Model file for the job. Use its own axes, mm. Round coordinates to 2 decimals unless told otherwise and drop trailing zeros. Loops run counter-clockwise (first coordinate to the right, second up) from the corner with the lowest first, then second, coordinate; pieces in that order, holes last. Notation, with made-up numbers: M -10,1 L 32,1 A12 ccw 32,22 Z; hole C -23.75,-29.5 d8. An arc over 180 degrees is marked long. Use a Markdown table: item, result. Add a question column.
Item 1: Saw through at B-B on y = -31. Write the cut outline in (x, z), then the cut area to 3 significant figures.
Item 2: Saw through at D-D on y = -20. Write the cut outline in (x, z).
Item 3: Saw through at A-A on x = 85.5. Write the cut outline in (y, z).
Item 4: Two-plate mould, pull along Y, no slides. Class faces 1 (the flat face through (11, 1, 2)), 2 (the cylindrical face through (81.73, 30.35, 0.99)): +Y half, -Y half, draft (parallel to the pull), parting line (faces both ways), or undercut.
Item 5: Saw through at C-C on z = 1.1. Write the cut outline in (x, y), then the cut area to 3 significant figures.
Item 6: Wall check: L1, parallel to Y at x = 79.5, z = 0.6; L2, parallel to Y at x = 72.5, z = 0.95; L3, parallel to X at y = -21.5, z = 0.8. Give the ranges that are in metal, low to high. Write a range as from..to.
Item 7: Pin check, flat tip, straight feed: P1, Ø4, axis at x = 29.68, y = 31, coming from the -Z side. Stop position of the tip, or through.
Autodesk Inventor part; units mm, degrees
ref_plane "YZ Plane" through (0, 0, 0) normal (1, 0, 0) x (0, 1, 0)
ref_plane "XZ Plane" through (0, 0, 0) normal (0, 1, 0) x (-1, 0, 0)
ref_plane "XY Plane" through (0, 0, 0) normal (0, 0, 1) x (1, 0, 0)
sketch "Sketch2" plane through (0, 0, 0) normal (0, 0, 1) x (1, 0, 0)
  line L0 (-40.3214, -37) -> (93.6786, -37)
  line L1 (93.6786, -37) -> (93.6786, -25)
  line L2 (93.6786, -25) -> (21.6786, -25)
  line L3 (19.6786, -23) -> (19.6786, 23)
  line L4 (21.6786, 25) -> (93.6786, 25)
  line L5 (93.6786, 25) -> (93.6786, 37)
  line L6 (93.6786, 37) -> (-40.3214, 37)
  line L7 (-40.3214, 37) -> (-40.3214, -37)
  arc A0 (21.6786, 25) -> (19.6786, 23) centre (21.6786, 23) ccw
  arc A1 (19.6786, -23) -> (21.6786, -25) centre (21.6786, -23) ccw
  circle A2 centre (-34.3214, 26) radius 2.15
  circle A3 centre (-34.3214, -26) radius 2.15
  circle A4 centre (29.6786, 31) radius 2.15
  circle A5 centre (79.6786, 31) radius 2.15
  circle A6 centre (79.6786, -31) radius 2.15
  circle A7 centre (29.6786, -31) radius 2.15
  point P0 (0, 0)
  dimension "d39" = 74
  dimension "d42" = 37
  dimension "d43" = 50
  dimension "d44" = 25
  dimension "d45" = 60
  dimension "d46" = 74
  dimension "d47" = 74
  dimension "d48" = 11
  dimension "d49" = 11
  dimension "d50" = 6
  dimension "d51" = 6
  dimension "d52" = 6
  dimension "d53" = 6
  dimension "d54" = 6
  dimension "d55" = 6
  dimension "d56" = 14
  dimension "d57" = 64
  dimension "d58" = 64
  dimension "d59" = 14
  dimension "d60" = 2
  dimension "d61" = 4.3
  dimension "d62" = 4.3
  dimension "d63" = 4.3
  dimension "d64" = 4.3
  dimension "d65" = 4.3
  dimension "d66" = 4.3
  dimension "d69" = 52
  dimension "d70" = 134
extrude "Extrusion4" add sketch "Sketch2" along normal blind 2
equation "\"d62\" = d61"
equation "\"d63\" = d61"
equation "\"d64\" = d61"
equation "\"d65\" = d61"
equation "\"d66\" = d61"
properties part number "top support extension"
Entries:
| question | item | result |
|---|---|---|
| 1 | outline | M -40.32,0 L 27.53,0 L 27.53,2 L -40.32,2 Z; M 31.83,0 L 77.53,0 L 77.53,2 L 31.83,2 Z; M 81.83,0 L 93.68,0 L 93.68,2 L 81.83,2 Z |
| 1 | area | 251 mm2 |
| 2 | outline | M -40.32,0 L 19.68,0 L 19.68,2 L -40.32,2 Z |
| 3 | outline | M -37,0 L -25,0 L -25,2 L -37,2 Z; M 25,0 L 37,0 L 37,2 L 25,2 Z |
| 4 | face 1 | draft |
| 4 | face 2 | undercut |
| 5 | outline | M -40.32,-37 L 93.68,-37 L 93.68,-25 L 21.68,-25 A2 cw 19.68,-23 L 19.68,23 A2 cw 21.68,25 L 93.68,25 L 93.68,37 L -40.32,37 Z; hole C -34.32,-26 d4.3; hole C -34.32,26 d4.3; hole C 29.68,-31 d4.3; hole C 29.68,31 d4.3; hole C 79.68,-31 d4.3; hole C 79.68,31 d4.3 |
| 5 | area | 6,130 mm2 |
| 6 | L1 | -37..-33.14, -28.86..-25, 25..28.86, 33.14..37 |
| 6 | L2 | -37..-25, 25..37 |
| 6 | L3 | -40.32..19.68 |
| 7 | P1 | through |
